```python
from build123d import *

# Parameters (mm, degrees)
SKETCH1_R    = 3.5
HEAD_DEPTH   = 4
SHANK_START  = -10
SKETCH2_R    = 2
SHANK_DEPTH  = 10
SOCKET_START = 4
SKETCH3_R    = 1.7
SOCKET_DEPTH = 2.4


with BuildPart() as part:
    # Sketch1 → Head (new body)
    with BuildSketch(Plane(origin=(0, 0, 0), x_dir=(1, 0, 0), z_dir=(0, 1, 0))):
        with Locations(Location((0, 0, 0), (0, 0, 270))):
            Circle(SKETCH1_R)
    extrude(amount=HEAD_DEPTH)

    # Sketch2 → Shank (add)
    with BuildSketch(Plane(origin=(0, 0, 0), x_dir=(1, 0, 0), z_dir=(0, 1, 0)).offset(SHANK_START)):
        with Locations(Location((0, 0, 0), (0, 0, 270))):
            Circle(SKETCH2_R)
    extrude(amount=SHANK_DEPTH)

    # Sketch3 → Socket (cut)
    with BuildSketch(Plane(origin=(0, 0, 0), x_dir=(1, 0, 0), z_dir=(0, 1, 0)).offset(SOCKET_START)):
        with Locations(Location((0, 0, 0), (0, 0, 270))):
            Circle(SKETCH3_R)
    extrude(amount=-SOCKET_DEPTH, mode=Mode.SUBTRACT)


solid = part.part
```
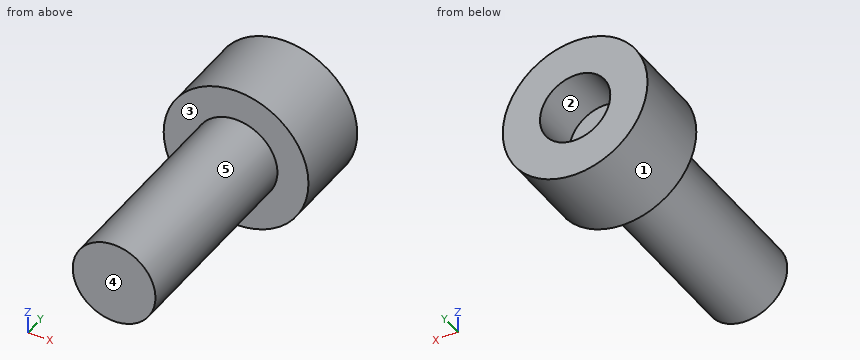
Can you work these out from the model? Positions are in its coordinate system, mm. Face numbers are marked on the shaded views. A direction names the side the tool comes from. Coordinates: 2 decimals unless noted, no trailing zeros. Loops run counter-clockwise (first coordinate to the right, second up) from the corner with the lowest first, then second, coordinate; pieces in that order, holes last. Notation, with made-up numbers: (-30, 61) - (-11, 61) arc R21 cw to (-11, 95) - close; hole circle Ø9 at (56.25, 54). An arc over 180 degrees is marked (long way). Answer as CSV lines item,"result". Start each with the question number.
1) Suppose I cut it at B-B (z = 0). Please give me the cut outline in (x, y), plus the area to 3 significant figures.
2) Thinking about a two-plate mould opening in Z: for the marked faces 1, 2 and 3, which applies, pulls with the +Z half, pulls with the -Z half, needs draft (parallel to the pull), parting line crosses it, or undercut?
3) Suppose I cut it at A-A (x = 0). Please give me the cut outline in (y, z).
4) For pin 1 (1.7 mm diameter, centred on x = -0.5, z = 0, fed in from +Y); pin 2 (1.5 mm diameter, centred on y = 2, z = -2, fed in from -X); pin 3 (3 mm diameter, centred on x = 0, y = -2.5, fed in from +Z), each with a flat end and sliding along its axis, tell me the tip position at first contact or that it passes through.
5) Which directions (+Z, -Z, +X, -X, +Y, -Y) give clear straight access to the entire face, cutting with the end or side of a thin tool? Please do the marked faces 4 and 5.
6) I need wall thicknesses on line 1 (X direction, y = 2.5, z = 0); line 2 (Y direction, x = 1.25, z = 2); line 3 (Y direction, x = -1, z = -0.5). Which ranges of each line are inside material? Lowest first, please. Write a range as from..to.
Check result:
1,outline,"(-3.5, 0) - (-2, 0) - (-2, -10) - (2, -10) - (2, 0) - (3.5, 0) - (3.5, 4) - (1.7, 4) - (1.7, 1.6) - (-1.7, 1.6) - (-1.7, 4) - (-3.5, 4) - close"
1,area,"59.8 mm²"
2,face 1,"parting line crosses it"
2,face 2,"undercut"
2,face 3,"needs draft"
3,outline,"(-10, -2) - (0, -2) - (0, -3.5) - (4, -3.5) - (4, -1.7) - (1.6, -1.7) - (1.6, 1.7) - (4, 1.7) - (4, 3.5) - (0, 3.5) - (0, 2) - (-10, 2) - close"
4,pin 1,"stops at y = 1.6"
4,pin 2,"stops at x = -3.27"
4,pin 3,"stops at z = 2"
5,face 4,"+Z, -Z, +X, -X, -Y"
5,face 5,"-Y"
6,line 1,"x = -3.5..-1.7, 1.7..3.5"
6,line 2,"y = 0..4"
6,line 3,"y = -10..1.6"
